Geometry: final body of the model. Coordinates: model frame, mm. A direction names the side the tool comes from. Round coordinates to 2 decimals unless told otherwise and drop trailing zeros. Loops run counter-clockwise (first coordinate to the right, second up) from the corner with the lowest first, then second, coordinate; pieces in that order, holes last. Notation, with made-up numbers: M 6.25,78 L 21.25,78 A24 cw 21.25,112 Z; hole C 36,36.5 d8. An arc over 180 degrees is marked long. Answer as a JSON object with one key per item and string values.
from build123d import *

# Parameters (mm, degrees)
SKETCH002_W  = 165
SKETCH002_H  = 200
PAD_DEPTH    = 80
THICKNESS_T  = 3
PAD004_DEPTH = 80


with BuildPart() as part:
    # Sketch002 → Pad (new body)
    with BuildSketch(Plane.XY):
        Rectangle(SKETCH002_W, SKETCH002_H)
    extrude(amount=PAD_DEPTH)

    # Thickness
    thickness_openings = [part.faces().sort_by_distance(p)[0] for p in [
        (0, 0, 80),
    ]]
    offset(amount=THICKNESS_T, openings=thickness_openings)

    # Sketch006 → Pad004 (join)
    with BuildSketch(Plane.XY.offset(80)):
        with BuildLine():
            ThreePointArc((-82.5, 95), (-78.964466, 96.464466), (-77.5, 100))
            Line((-82.5, 100), (-77.5, 100))
            Line((-82.5, 95), (-82.5, 100))
        make_face()
        with BuildLine():
            ThreePointArc((77.5, 100), (78.964466, 96.464466), (82.5, 95))
            Line((82.5, 100), (82.5, 95))
            Line((82.5, 100), (77.5, 100))
        make_face()
        with BuildLine():
            ThreePointArc((-77.5, -100), (-78.964466, -96.464466), (-82.5, -95))
            Line((-82.5, -100), (-82.5, -95))
            Line((-82.5, -100), (-77.5, -100))
        make_face()
        with BuildLine():
            ThreePointArc((82.5, -95), (78.964466, -96.464466), (77.5, -100))
            Line((77.5, -100), (82.5, -100))
            Line((82.5, -100), (82.5, -95))
        make_face()
        with BuildLine():
            ThreePointArc((5, -100), (0, -95), (-5, -100))
            Line((-5, -100), (5, -100))
        make_face()
        with BuildLine():
            ThreePointArc((-82.5, -5), (-77.5, 0), (-82.5, 5))
            Line((-82.5, 5), (-82.5, -5))
        make_face()
        with BuildLine():
            ThreePointArc((82.5, 5), (77.5, 0), (82.5, -5))
            Line((82.5, 5), (82.5, -5))
        make_face()
        with BuildLine():
            ThreePointArc((-5, 100), (0, 95), (5, 100))
            Line((-5, 100), (5, 100))
        make_face()
    extrude(amount=-PAD004_DEPTH)


solid = part.part
1) Section query C-C (z = 45). Return the cut outline in (x, y).
Results:
{"outline": "M -85.5,-100 A3 ccw -82.5,-103 L 82.5,-103 A3 ccw 85.5,-100 L 85.5,100 A3 ccw 82.5,103 L -82.5,103 A3 ccw -85.5,100 Z; hole M -82.5,-95 A5 cw -77.5,-100 L -5,-100 A5 cw 5,-100 L 77.5,-100 A5 cw 82.5,-95 L 82.5,-5 A5 cw 82.5,5 L 82.5,95 A5 cw 77.5,100 L 5,100 A5 cw -5,100 L -77.5,100 A5 cw -82.5,95 L -82.5,5 A5 cw -82.5,-5 Z"}
2) Section query A-A (x = 15). Return the cut outline in (y, z), and give its area (3 significant figures).
Results:
{"outline": "M -103,0 A3 ccw -100,-3 L 100,-3 A3 ccw 103,0 L 103,80 L 100,80 L 100,0 L -100,0 L -100,80 L -103,80 Z", "area": "1,090 mm2"}
3) Reachability of faces 1 (the flat face through (-1, 103, 39)), 2 (the flat face through (82.5, -51, 39)) from +Z, -Z, +X, -X, +Y, -Y: full face, straight path, thin tool, end or side. Return the list, or none.
Results:
{"face 1": "+Z, -Z, +X, -X, +Y", "face 2": "+Z"}
4) Pull-direction query (X, two-part tool) for faces 3 (the cylindrical face through (79, -96.43, 40.56)), 4 (the flat face through (-83, 0, 80)); classes: +X half, -X half, draft (parallel to the pull), parting line (faces both ways), or undercut.
Results:
{"face 3": "undercut", "face 4": "draft"}
5) Pin query (flat end, axial travel): P1, Ø10, axis at x = -21, y = -61.5, coming from the +Z side. Return the tip coordinate at first contact, or that it passes through.
Results:
{"P1": "z = 0"}
6) Ray query, line 1 (Y direction, x = 57, z = 9.5); line 2 (X direction, y = 63, z = 55); line 3 (Z direction, x = 24.5, y = 68). Return the intervals inside material, ascending.
Results:
{"line 1": "-103 to -100, 100 to 103", "line 2": "-85.5 to -82.5, 82.5 to 85.5", "line 3": "-3 to 0"}
7) Section query B-B (y = 0). Return the cut outline in (x, z).
Results:
{"outline": "M -85.5,0 A3 ccw -82.5,-3 L 82.5,-3 A3 ccw 85.5,0 L 85.5,80 L 77.5,80 L 77.5,0 L -77.5,0 L -77.5,80 L -85.5,80 Z"}
